Geometry: see drawing. Coordinates: mm, zero at the bounding-box minimum. Round coordinates to 2 decimals unless told otherwise and drop trailing zeros. Order: outer loops, then holes, each group sorted by start corner. A loop starts at its lowest first (then second) coordinate and runs counter-clockwise, first axis right, second up.
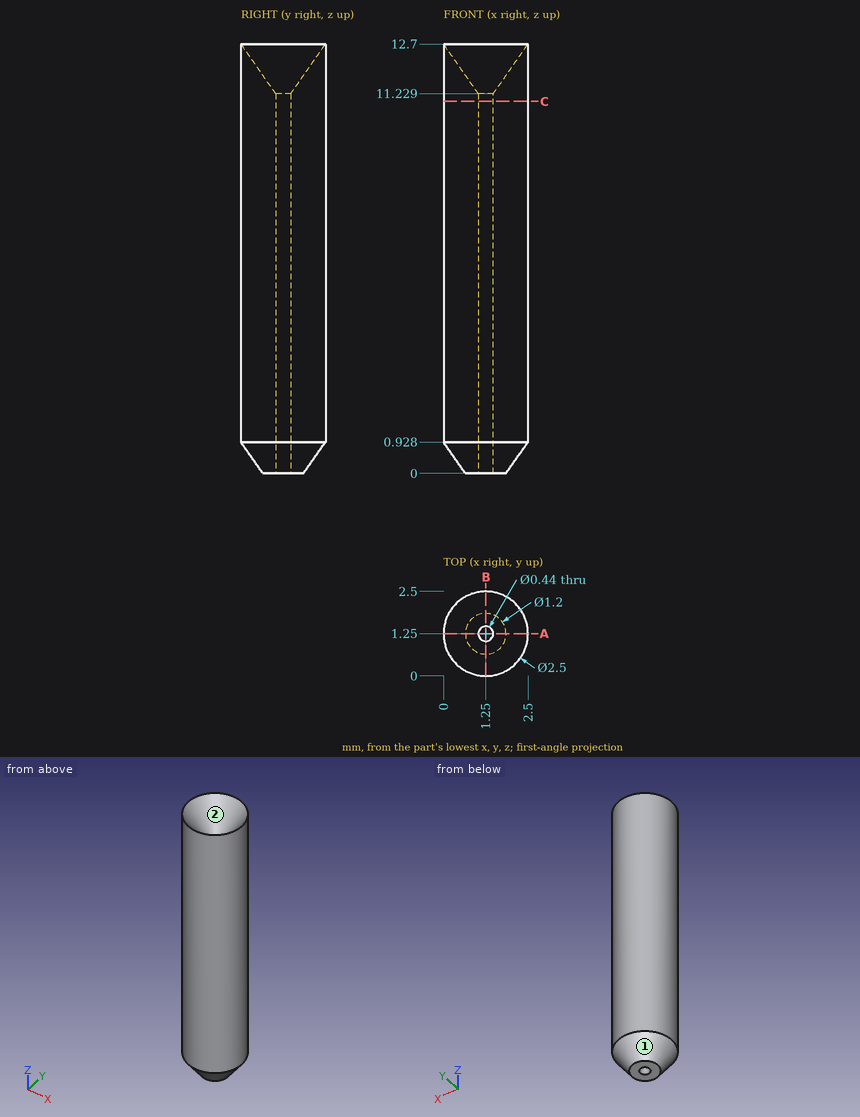
1. Pull-direction query (X, two-part tool) for the marked faces 1 and 2; classes: released by +X, released by -X, zero draft, split by the parting line, or undercut.
2. Section C-C on z = 11. Return loops of the section in (x, y).
3. Section A-A on y = 1.25. Return loops of the section in (x, z).
4. Line query: line 1 along Y through (x, z) = (1.25, 3.5); line 2 along X through (y, z) = (1.4, 4.25); line 3 along Y through (x, z) = (1.8, 12.25) (1 decimal). Output: solid intervals per line, ascending.
Result:
1. face 1: split by the parting line
1. face 2: undercut
2. outline: circle Ø2.5 at (1.25, 1.25); hole circle Ø0.44 at (1.25, 1.25)
3. outline: (0, 0.93) - (0.65, 0) - (1.03, 0) - (1.03, 11.23) - (0, 12.7) - close; (1.47, 0) - (1.85, 0) - (2.5, 0.93) - (2.5, 12.7) - (1.47, 11.23) - close
4. line 1: y = 0 to 1.03, 1.47 to 2.5
4. line 2: x = 0.01 to 1.09, 1.41 to 2.49
4. line 3: y = 0.1 to 0.5, 2 to 2.4
